Build history of the part. All positions in model axes, mm. Face numbers are marked on the shaded views. Round coordinates to 2 decimals unless told otherwise and drop trailing zeros. Loops run counter-clockwise (first coordinate to the right, second up) from the corner with the lowest first, then second, coordinate; pieces in that order, holes last. Notation, with made-up numbers: (60.5, 39.5) -> (113.5, 39.5) arc R26 cw to (113.5, 65.5) -> close; hole circle Ø10 at (-35.75, 53.25). An arc over 180 degrees is marked (long way). Put each result on its own line as item: value. Start each with the question number.
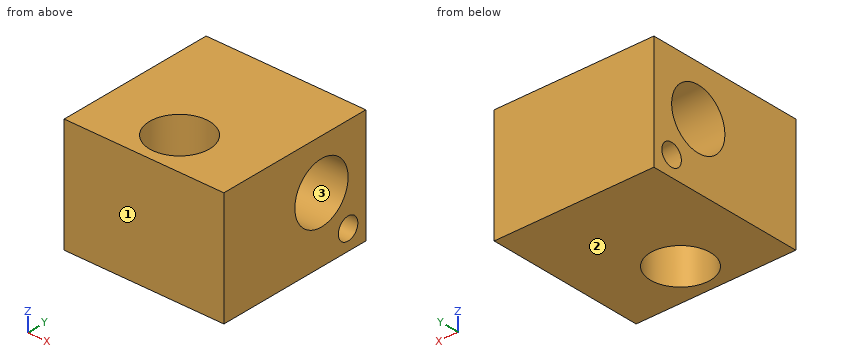
```python
from build123d import *

# Parameters (mm, degrees)
F0_W     = 16
F0_H     = 16
F1_DEPTH = 11.5
F2_R     = 3
F3_DEPTH = 25
F4_R     = 3
F4_R_2   = 1.1
F5_DEPTH = 16.001


with BuildPart() as f1:
    # F0 (on Top) → F1 (new body)
    with BuildSketch(Plane.XY):
        Rectangle(F0_W, F0_H)
    extrude(amount=F1_DEPTH)

    # F2 (on face) → F3 (cut)
    with BuildSketch(Plane.XY.offset(11.5)):
        with Locations((0, -4)):
            Circle(F2_R)
    extrude(amount=-F3_DEPTH, mode=Mode.SUBTRACT)

    # F4 (on face) → F5 (cut, through all)
    with BuildSketch(Plane.YZ.offset(8)):
        with Locations((3, 6.5)):
            Circle(F4_R)
        with Locations((6, 2)):
            Circle(F4_R_2)
    extrude(amount=-F5_DEPTH, mode=Mode.SUBTRACT)


solid = f1.part
```
Item 1: Cut at A-A on z = 6.5. Write the cut outline in (x, y).
Item 2: Cut at C-C on x = 0. Write the cut outline in (y, z).
Item 3: Pull direction Y, two halves, no side cores. Call the marked faces 1, 2 and 3: +Y half, -Y half, draft (parallel to the pull), parting line (faces both ways), or undercut.
Item 4: Wall check: line 1 (Y direction, x = 0, z = 5.25); line 2 (Y direction, x = 2.5, z = 5); line 3 (Z direction, x = 2, y = 3). Give the ranges that are in metal, low to high. Write a range as from..to.
Item 5: Cut at D-D on x = 3.25. Write the cut outline in (y, z), then the cut area to 3 significant figures.
Item 6: Cut at B-B on y = 3. Write the cut outline in (x, z), then the cut area to 3 significant figures.
Ans:
1. outline: (-8, -8) -> (8, -8) -> (8, 0) -> (-8, 0) -> close; (-8, 6) -> (8, 6) -> (8, 8) -> (-8, 8) -> close; hole circle Ø6 at (0, -4)
2. outline: (-8, 0) -> (-7, 0) -> (-7, 11.5) -> (-8, 11.5) -> close; (-1, 0) -> (8, 0) -> (8, 11.5) -> (-1, 11.5) -> close; hole circle Ø6 at (3, 6.5); hole circle Ø2.2 at (6, 2)
3. face 1: -Y half
3. face 2: draft
3. face 3: undercut
4. line 1: y = -8..-7, -1..0.27, 5.73..8
4. line 2: y = -8..-5.66, -2.34..0.4, 5.6..8
4. line 3: z = 0..3.5, 9.5..11.5
5. outline: (-8, 0) -> (8, 0) -> (8, 11.5) -> (-8, 11.5) -> close; hole circle Ø6 at (3, 6.5); hole circle Ø2.2 at (6, 2)
5. area: 152 mm2
6. outline: (-8, 0) -> (8, 0) -> (8, 3.5) -> (-8, 3.5) -> close; (-8, 9.5) -> (8, 9.5) -> (8, 11.5) -> (-8, 11.5) -> close
6. area: 88.0 mm2
